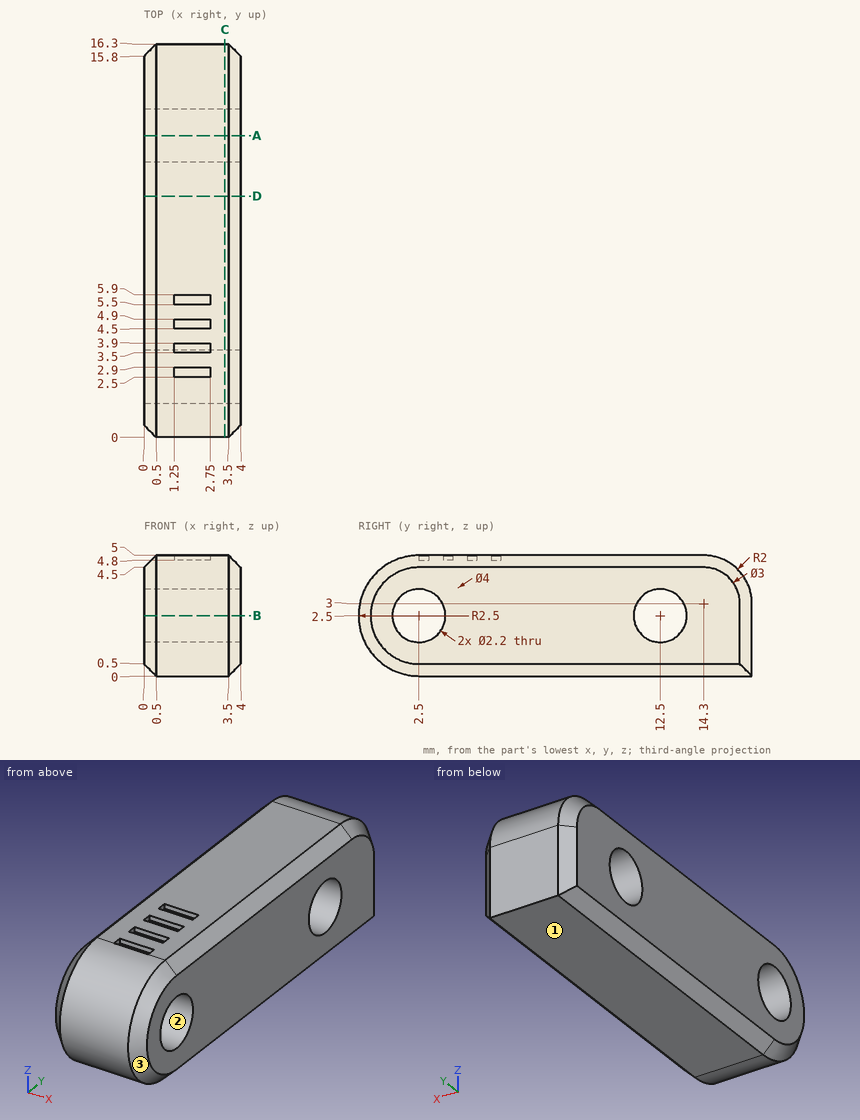
Study the drawing (mm; zero at the part's minimum x, y, z) and answer. Round coordinates to 2 decimals unless told otherwise and drop trailing zeros. Order: outer loops, then holes, each group sorted by start corner. A loop starts at its lowest first (then second) coordinate and runs counter-clockwise, first axis right, second up. Notation, with made-up numbers: (69.25, -3) - (98.25, -3) arc R14 ccw to (98.25, 5) - close; hole circle Ø11 at (45, 51.5). An arc over 180 degrees is marked (long way). Use one line per item in the form item = value. Start each with the question number.
(1) The part is cut by section C-C (x = 3.35). Give the vertices of the cut face in (y, z), then the cut area to 3 significant figures.
(2) Find the intervals of material crossed by line 1 along Y through (x, z) = (1.6, 3.5); line 2 along Y through (x, z) = (1.7, 2.4); line 3 along Z through (x, y) = (3.05, 2.5), in increasing order. Write a range as from..to.
(3) A flat-ended cylindrical pin translates along its axis: pin 1 Ø1.8 at (y, z) = (2.5, 2.5) entering from -X. Find the tip coordinate at first contact, or state that the pin passes through.
(4) The part is cut by section B-B (z = 2.5). Give the vertices of the cut face in (x, y).
(5) The part is cut by section D-D (y = 10). Give the vertices of the cut face in (x, z).
(6) The part is cut by section A-A (y = 12.5). Give the vertices of the cut face in (x, z).
(7) Determine the mould class of the marked faces 1, 2 and 3 for opening direction Y: +Y half, -Y half, draft (parallel to the pull), parting line (faces both ways), or undercut.
Checked values:
q1.outline = (2.5, 0) - (16.3, 0) - (16.3, 3) arc R2 ccw to (14.3, 5) - (2.5, 5) arc R2.5 ccw to start; hole circle Ø2.2 at (2.5, 2.5); hole circle Ø2.2 at (12.5, 2.5)
q1.area = 70.4 mm^2
q2.line_1 = 0.21..2.04, 2.96..12.04, 12.96..16.24
q2.line_2 = 0..1.4, 3.6..11.4, 13.6..16.3
q2.line_3 = 0..1.4, 3.6..5
q3.pin_1 = through
q4.outline = (0, 0.5) - (0.5, 0) - (3.5, 0) - (4, 0.5) - (4, 1.4) - (0, 1.4) - close; (0, 3.6) - (4, 3.6) - (4, 11.4) - (0, 11.4) - close; (0, 13.6) - (4, 13.6) - (4, 15.8) - (3.5, 16.3) - (0.5, 16.3) - (0, 15.8) - close
q5.outline = (0, 0.5) - (0.5, 0) - (3.5, 0) - (4, 0.5) - (4, 4.5) - (3.5, 5) - (0.5, 5) - (0, 4.5) - close
q6.outline = (0, 0.5) - (0.5, 0) - (3.5, 0) - (4, 0.5) - (4, 1.4) - (0, 1.4) - close; (0, 3.6) - (4, 3.6) - (4, 4.5) - (3.5, 5) - (0.5, 5) - (0, 4.5) - close
q7.face_1 = draft
q7.face_2 = undercut
q7.face_3 = -Y half
